from build123d import *

# Parameters (mm, degrees)
SKETCH1_W           = 37
SKETCH1_H           = 60
BOSS_EXTRUDE1_DEPTH = 3
CUT_EXTRUDE1_DEPTH  = 3
SKETCH3_W           = 3
SKETCH3_H           = 5
BOSS_EXTRUDE2_DEPTH = 3
SKETCH4_W           = 3
SKETCH4_H           = 5
BOSS_EXTRUDE3_DEPTH = 3


with BuildPart() as part:
    # Sketch1 → Boss-Extrude1 (new body)
    with BuildSketch(Plane(origin=(0, 0, 0), x_dir=(0, 0, -1), z_dir=(1, 0, 0))):
        Rectangle(SKETCH1_W, SKETCH1_H)
    extrude(amount=BOSS_EXTRUDE1_DEPTH)

    # Sketch2 → Cut-Extrude1 (cut)
    with BuildSketch(Plane(origin=(3, 0, 0), x_dir=(0, 0, -1), z_dir=(1, 0, 0))):
        Polygon((-18.5, -30), (18.5, 30), (-18.5, 30), align=None)
    extrude(amount=-CUT_EXTRUDE1_DEPTH, mode=Mode.SUBTRACT)

    # Sketch3 → Boss-Extrude2 (add)
    with BuildSketch(Plane.XZ.offset(30)):
        with Locations((1.5, 11)):
            Rectangle(SKETCH3_W, SKETCH3_H)
        with Locations((1.5, -11)):
            Rectangle(SKETCH3_W, SKETCH3_H)
    extrude(amount=BOSS_EXTRUDE2_DEPTH)

    # Sketch4 → Boss-Extrude3 (add)
    with BuildSketch(Plane(origin=(0, 0, -18.5), x_dir=(-1, 0, 0), z_dir=(0, 0, -1))):
        with Locations((-1.5, -22.5)):
            Rectangle(SKETCH4_W, SKETCH4_H)
        with Locations((-1.5, 22.5)):
            Rectangle(SKETCH4_W, SKETCH4_H)
    extrude(amount=BOSS_EXTRUDE3_DEPTH)


solid = part.part
The model under review builds one solid part; all positions refer to its coordinate system, in mm. A direction names the side the tool comes from. Give positions to 0.01 mm unless a question says otherwise; leave off trailing zeros. Loops run counter-clockwise (first coordinate to the right, second up) from the corner with the lowest first, then second, coordinate; pieces in that order, holes last. Notation, with made-up numbers: (-35.75, -18.75) -> (-18.75, -18.75) arc R11 cw to (-18.75, -9.75) -> close; hole circle Ø4 at (0, 13.25). An arc over 180 degrees is marked (long way). Answer as a JSON object with one key per item and string values. Group by question number.
Q1. Draft analysis for pull direction Y (two halves, no side actions). For faces 5 (the flat face through (1, -30, -16)), 6 (the flat face through (2, 20, -20)), 7 (the flat face through (1, 0, -18.5)), 8 (the flat face through (1, -31, -13.5)), state which applies: pulls with the +Y half, pulls with the -Y half, needs draft (parallel to the pull), parting line crosses it, or undercut.
Q2. Tool access review of faces 1 (the flat face through (1, -31, 13.5)), 2 (the flat face through (1, 27, -18.5)), 3 (the flat face through (1, -28, -18.5)), 4 (the flat face through (1, -31, 8.5)): name each direction out of +Z, -Z, +X, -X, +Y, -Y from which nothing blocks a thin tool from reaching the whole face with its end or side.
Q3. Wall thickness on line 1 along Z through (x, y) = (0.25, -8); line 2 along Z through (x, y) = (2.4, 22.5) (3 decimals); line 3 along Y through (x, z) = (0.35, -14): over which ranges is each line inside the solid? List them lowest first.
Q4. Take a section at C-C (z = 9.5). Write out the cut boundary in (x, y), plus the area to 3 significant figures.
Q5. Take a section at B-B (y = -12). Write out the cut boundary in (x, z).
Q6. Insertion check: pin 1 (0.9 mm diameter, centred on x = 2, z = -17, fed in from -Y); pin 2 (0.9 mm diameter, centred on x = 2, y = -6.5, fed in from -Z); pin 3 (1.5 mm diameter, centred on x = 1.5, y = -31, fed in from -Z). Each pin has a flat end and moves straight along its axis. Give the tip position at first contact, or say it passes through.
Q7. Take a section at A-A (x = 2.4). Write out the cut boundary in (y, z).
Answer below:
{
 "1": {"face 5": "pulls with the -Y half", "face 6": "undercut", "face 7": "undercut", "face 8": "needs draft"},
 "2": {"face 1": "+Z, +X, -X, -Y", "face 2": "-Z, +X, -X, +Y", "face 3": "-Z, +X, -X, -Y", "face 4": "+X, -X, -Y"},
 "3": {"line 1": "z = -18.5 to 4.93", "line 2": "z = -21.5 to -13.875", "line 3": "y = -30 to 22.7"},
 "4": {"outline": "(0, -33) -> (3, -33) -> (3, -15.41) -> (0, -15.41) -> close", "area": "52.8 mm2"},
 "5": {"outline": "(0, -18.5) -> (3, -18.5) -> (3, 7.4) -> (0, 7.4) -> close"},
 "6": {"pin 1": "stops at y = -30", "pin 2": "stops at z = -18.5", "pin 3": "stops at z = -13.5"},
 "7": {"outline": "(-33, -13.5) -> (-30, -13.5) -> (-30, -18.5) -> (-25, -18.5) -> (-25, -21.5) -> (-20, -21.5) -> (-20, -18.5) -> (20, -18.5) -> (20, -21.5) -> (25, -21.5) -> (25, -18.5) -> (30, -18.5) -> (-30, 18.5) -> (-30, 13.5) -> (-33, 13.5) -> (-33, 8.5) -> (-30, 8.5) -> (-30, -8.5) -> (-33, -8.5) -> close"}
}
